Geometry: final body of the model. Coordinates: model frame, mm. A direction names the side the tool comes from. Coordinates: 2 decimals unless noted, no trailing zeros. Write each loop counter-clockwise with the first axis right and the second up, starting at its lowest first coordinate (ties: lowest second). Pieces come first, ordered by that corner, then holes. Notation, with made-up numbers: (-36, 14.5) -> (13, 14.5) arc R24 ccw to (13, 34.5) -> close; hole circle Ø6 at (40.5, 3.25). An arc over 180 degrees is marked (long way). One line per item, written item: value.
```python
from build123d import *

# Parameters (mm, degrees)
SKETCH1_W           = 12
SKETCH1_H           = 12
BOSS_EXTRUDE1_DEPTH = 4.3
SKETCH2_W           = 3.8
SKETCH2_H           = 3.8
BOSS_EXTRUDE2_DEPTH = 3
SKETCH3_W           = 106
SKETCH3_H           = 36
SKETCH3_R           = 2
BOSS_EXTRUDE3_DEPTH = 1.6
SKETCH4_W           = 12
SKETCH4_H           = 12
BOSS_EXTRUDE4_DEPTH = 4.3
SKETCH5_W           = 3.8
SKETCH5_H           = 3.8
BOSS_EXTRUDE5_DEPTH = 3


with BuildPart() as part:
    # Sketch1 → Boss-Extrude1 (new body)
    with BuildSketch(Plane(origin=(0, 0, 0), x_dir=(1, 0, 0), z_dir=(0, 1, 0))):
        with Locations((6, 6)):
            Rectangle(SKETCH1_W, SKETCH1_H)
    extrude(amount=BOSS_EXTRUDE1_DEPTH)

    # Sketch2 → Boss-Extrude2 (add)
    with BuildSketch(Plane(origin=(0, 4.3, 0), x_dir=(1, 0, 0), z_dir=(0, 1, 0))):
        with Locations((6, 6)):
            Rectangle(SKETCH2_W, SKETCH2_H)
    extrude(amount=BOSS_EXTRUDE2_DEPTH)

    # Sketch3 → Boss-Extrude3 (add)
    with BuildSketch(Plane.XZ):
        with Locations((41, -6)):
            Rectangle(SKETCH3_W, SKETCH3_H)
        with Locations(Location((-8, -20, 0), (0, 0, 270))):
            Circle(SKETCH3_R, mode=Mode.SUBTRACT)
        with Locations(Location((-8, 8, 0), (0, 0, 270))):
            Circle(SKETCH3_R, mode=Mode.SUBTRACT)
        with Locations(Location((90, 8, 0), (0, 0, 270))):
            Circle(SKETCH3_R, mode=Mode.SUBTRACT)
        with Locations(Location((90, -20, 0), (0, 0, 270))):
            Circle(SKETCH3_R, mode=Mode.SUBTRACT)
    extrude(amount=BOSS_EXTRUDE3_DEPTH)

    # Sketch4 → Boss-Extrude4 (add)
    with BuildSketch(Plane(origin=(0, 0, 0), x_dir=(1, 0, 0), z_dir=(0, 1, 0))):
        with Locations((41, 6)):
            Rectangle(SKETCH4_W, SKETCH4_H)
        with Locations((76, 6)):
            Rectangle(SKETCH4_W, SKETCH4_H)
    extrude(amount=BOSS_EXTRUDE4_DEPTH)

    # Sketch5 → Boss-Extrude5 (add)
    with BuildSketch(Plane(origin=(0, 4.3, 0), x_dir=(1, 0, 0), z_dir=(0, 1, 0))):
        with Locations((41, 6)):
            Rectangle(SKETCH5_W, SKETCH5_H)
        with Locations((76, 6)):
            Rectangle(SKETCH5_W, SKETCH5_H)
    extrude(amount=BOSS_EXTRUDE5_DEPTH)


solid = part.part
```
(1) First-contact query: pin 1 (1.3 mm diameter, centred on y = 3, z = -5.5, fed in from -X); pin 2 (1.5 mm diameter, centred on y = 5.5, z = -6, fed in from +X); pin 3 (2 mm diameter, centred on x = 40.5, y = 1.5, fed in from +Z); pin 4 (1.5 mm diameter, centred on x = 50.5, y = 2.5, fed in from -Z). Flat tips, straight axial feed; report the tip coordinate or a pass-through.
Responses:
pin 1: stops at x = 0
pin 2: stops at x = 77.9
pin 3: stops at z = 0
pin 4: passes through
(2) Section C-C (x = 50.5). Return the cut outline in (y, z), then the cut area to 3 significant figures.
Responses:
outline: (-1.6, -24) -> (0, -24) -> (0, 12) -> (-1.6, 12) -> close
area: 57.6 mm2
(3) Pull-direction query (Z, two-part tool) for faces 5 (the cylindrical face through (92, -1, -20)), 6 (the flat face through (39.1, 6, -6)), 7 (the flat face through (41, 6, -4.1)); classes: released by +Z, released by -Z, zero draft, split by the parting line, or undercut.
Responses:
face 5: undercut
face 6: zero draft
face 7: released by +Z
(4) Reachability of faces 1 (the flat face through (6, 2, -12)), 2 (the flat face through (6, 2, 0)), 3 (the flat face through (82, 2, -6)), 4 (the flat face through (47, 2, -6)) from +Z, -Z, +X, -X, +Y, -Y: full face, straight path, thin tool, end or side. Return the list, or none.
Responses:
face 1: -Z, +X, -X, +Y
face 2: +Z, +X, -X, +Y
face 3: +Z, -Z, +X, +Y
face 4: +Z, -Z, +Y
(5) Line query: line 1 (X direction, y = -0.6, z = -20); line 2 (X direction, y = 5, z = -6); line 3 (Y direction, x = 0.5, z = 7). Output: solid intervals per line, ascending. Write a range as [from, to].
Responses:
line 1: x = [-12, -10], [-6, 88], [92, 94]
line 2: x = [4.1, 7.9], [39.1, 42.9], [74.1, 77.9]
line 3: y = [-1.6, 0]
(6) Section B-B (y = 5.75). Return the cut outline in (x, z), then the cut area to 3 significant figures.
Responses:
outline: (4.1, -7.9) -> (7.9, -7.9) -> (7.9, -4.1) -> (4.1, -4.1) -> close; (39.1, -7.9) -> (42.9, -7.9) -> (42.9, -4.1) -> (39.1, -4.1) -> close; (74.1, -7.9) -> (77.9, -7.9) -> (77.9, -4.1) -> (74.1, -4.1) -> close
area: 43.3 mm2
(7) Section A-A (z = -20). Return the cut outline in (x, y), then the cut area to 3 significant figures.
Responses:
outline: (-12, -1.6) -> (-10, -1.6) -> (-10, 0) -> (-12, 0) -> close; (-6, -1.6) -> (88, -1.6) -> (88, 0) -> (-6, 0) -> close; (92, -1.6) -> (94, -1.6) -> (94, 0) -> (92, 0) -> close
area: 157 mm2
